Model file for the job. Use its own axes, mm. Face numbers are marked on the shaded views. A direction names the side the tool comes from. Coordinates: 2 decimals unless noted, no trailing zeros. Order: outer loops, then holes, each group sorted by start corner. A loop starts at its lowest first (then second) coordinate and runs counter-clockwise, first axis right, second up. Notation, with made-up numbers: (81, -27) -> (87, -27) arc R7 cw to (87, -17) -> close; hole circle Ø2 at (73.5, -14). An arc over 180 degrees is marked (long way). Return JSON: item names as keys, results as strings. Group by question number.
1) Which spindle directions (+Z, -Z, +X, -X, +Y, -Y) get a long thin tool onto all of the face, cutting with end or side? Do the marked faces 4 and 5. Say none if no direction does.
2) Cut at D-D (y = 73). Write the cut outline in (x, z), and give its area (3 significant figures).
3) Cut at B-B (x = 12). Write the cut outline in (y, z).
4) Pull direction Y, two halves, no side cores. Call the marked faces 1, 2 and 3: +Y half, -Y half, draft (parallel to the pull), parting line (faces both ways), or undercut.
5) Flat gauge pins, fed straight in: pin 1 (10 mm diameter, centred on y = 12, z = 16, fed in from -X); pin 2 (1 mm diameter, centred on x = 37.5, y = 57, fed in from -Z); pin 3 (5.5 mm diameter, centred on x = 11, y = 41.5, fed in from +Z). Where does each tip first touch, or does it go through?
6) Cut at A-A (z = 17.5). State how many separate pieces and enclosed holes the cut face has, and give its area (3 significant figures).
7) Probe line 1 (X direction, y = 26, z = 20.5); line 2 (Y direction, x = 53, z = 32.5); line 3 (X direction, y = 51.5, z = 6). List the from-to ranges inside material, lowest first.
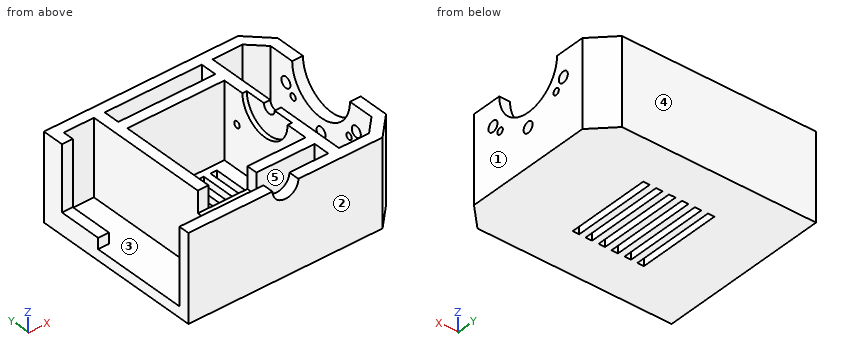
Autodesk Inventor part; units mm, degrees
ref_plane "YZ Plane" through (0, 0, 0) normal (1, 0, 0) x (0, 1, 0)
ref_plane "XZ Plane" through (0, 0, 0) normal (0, 1, 0) x (-1, 0, 0)
ref_plane "XY Plane" through (0, 0, 0) normal (0, 0, 1) x (1, 0, 0)
sketch "Sketch1" plane through (0, 0, 0) normal (0, 0, 1) x (1, 0, 0)
  line L0 (0, 0) -> (100, 0)
  line L1 (100, 0) -> (100, 80) construction
  line L2 (100, 80) -> (0, 80)
  line L3 (0, 80) -> (0, 0)
  line L4 (100, 70) -> (90, 80)
  line L5 (100, 10) -> (90, 0)
  line L6 (100, 70) -> (100, 10)
  line L7 (90, 0) -> (0, 0)
  line L8 (90, 80) -> (0, 80)
  dimension "d0" = 100
  dimension "d1" = 80
  dimension "d15" = 10
  dimension "d16" = 10
  dimension "d17" = 10
  dimension "d18" = 10
extrude "Extrusion1" add sketch "Sketch1" along normal blind 40
sketch "Sketch2" plane through (0, 0, 40) normal (0, 0, 1) x (1, 0, 0)
  line L0 (90, 80) -> (0, 80)
  line L1 (100, 70) -> (90, 80)
  line L2 (100, 10) -> (100, 70)
  line L3 (90, 0) -> (100, 10)
  line L4 (0, 0) -> (90, 0)
  line L5 (0, 75) -> (87.9289, 75)
  line L6 (87.9289, 75) -> (95, 67.9289)
  line L7 (95, 67.9289) -> (95, 12.0711)
  line L8 (95, 12.0711) -> (87.9289, 5)
  line L9 (87.9289, 5) -> (0, 5)
  line L10 (0, 80) -> (0, 0)
  line L11 (0, 75) -> (0, 5)
  dimension "d19" = 5
extrude "Extrusion2" cut sketch "Sketch2" against normal blind 35 contours L5 L6 L7 L8 L9 L10
sketch "Sketch3" plane through (0, 0, 0) normal (-1, 0, 0) x (0, 0, 1)
  line L0 (0, 80) -> (40, 80)
  line L1 (0, 0) -> (40, 0)
  line L2 (0, 80) -> (10, 80)
  line L3 (10, 80) -> (10, 50)
  line L4 (10, 50) -> (0, 50)
  line L5 (0, 50) -> (0, 80)
  line L6 (40, 80) -> (40, 0)
  line L7 (0, 80) -> (40, 80)
  line L8 (40, 80) -> (40, 70)
  line L9 (40, 70) -> (0, 70)
  line L10 (0, 70) -> (0, 80)
  line L11 (0, 0) -> (40, 0)
  line L12 (0, 80) -> (40, 80)
  point P0 (20, 0)
  point P1 (20, 80)
  dimension "d7" = 10
  dimension "d8" = 10
  dimension "d11" = 50
extrude "Extrusion3" add sketch "Sketch3" against normal blind 5
sketch "Sketch4" plane through (100, 10, 0) normal (1, 0, 0) x (0, 0, -1)
  circle A0 centre (-40, 30) radius 16
  line L0 (-40, 0) -> (-40, 60)
  point P0 (66.6667, -50)
  dimension "d12" = 32
extrude "Extrusion4" cut sketch "Sketch4" against normal through all
sketch "Sketch5" plane through (0, 0, 5) normal (0, 0, 1) x (1, 0, 0)
  line L0 (74, 75) -> (69, 75)
  line L1 (69, 75) -> (69, 5)
  line L2 (69, 5) -> (74, 5)
  line L3 (74, 5) -> (74, 75)
  line L4 (87.9289, 5) -> (0, 5)
  line L5 (5, 75) -> (87.9289, 75)
  line L6 (95, 67.9289) -> (95, 56)
  point P0 (0, 0)
  dimension "d20" = 5
  dimension "d21" = 21
extrude "Extrusion5" add sketch "Sketch5" along normal blind 35
sketch "Sketch6" plane through (69, 5, 5) normal (-1, 0, 0) x (0, 0, 1)
  line L0 (35, 70) -> (35, 0)
  circle A0 centre (35, 35) radius 3
  line L1 (19.5, 19.5) -> (50.5, 19.5) construction
  line L2 (50.5, 19.5) -> (50.5, 50.5) construction
  line L3 (50.5, 50.5) -> (19.5, 50.5) construction
  line L4 (19.5, 50.5) -> (19.5, 19.5) construction
  line L5 (19.5, 19.5) -> (50.5, 50.5) construction
  line L6 (50.5, 19.5) -> (19.5, 50.5) construction
  circle A1 centre (19.5, 50.5) radius 1.5
  circle A2 centre (19.5, 19.5) radius 1.5
  point P0 (-5, -5)
  dimension "d24" = 6
  dimension "d25" = 31
  dimension "d26" = 31
  dimension "d27" = 3
  dimension "d28" = 3
extrude "Extrusion6" cut sketch "Sketch6" against normal through all
sketch "Sketch7" plane through (69, 5, 5) normal (-1, 0, 0) x (0, 0, 1)
  arc A0 (35, 38) -> (35, 32) centre (35, 35) ccw
  circle A1 centre (35, 35) radius 12.5
  point P0 (-5, -5)
  dimension "d31" = 25
extrude "Extrusion7" cut sketch "Sketch7" against normal blind 2
sketch "Sketch8" plane through (0, 0, 5) normal (0, 0, 1) x (1, 0, 0)
  line L0 (69, 17.5) -> (19, 17.5)
  line L1 (19, 17.5) -> (19, 12.5)
  line L2 (19, 12.5) -> (69, 12.5)
  line L3 (69, 12.5) -> (69, 17.5)
  line L4 (69, 27.5) -> (69, 5)
  line L5 (69, 67.5) -> (19, 67.5)
  line L6 (19, 67.5) -> (19, 62.5)
  line L7 (19, 62.5) -> (69, 62.5)
  line L8 (69, 62.5) -> (69, 67.5)
  line L9 (19, 62.5) -> (19, 17.5) construction
  line L10 (69, 27.5) -> (69, 52.5) construction
  point P0 (0, 0)
  point P1 (69, 15)
  point P2 (19, 40)
  point P3 (69, 40)
  dimension "d34" = 50
  dimension "d35" = 5
  dimension "d36" = 50
  dimension "d37" = 5
  dimension "d38" = 45
extrude "Extrusion8" add sketch "Sketch8" along normal blind 35
sketch "Sketch9" plane through (0, 0, 5) normal (0, 0, 1) x (1, 0, 0)
  line L0 (19, 75) -> (24, 75)
  line L1 (24, 75) -> (24, 5)
  line L2 (24, 5) -> (19, 5)
  line L3 (19, 5) -> (19, 75)
  line L4 (5, 75) -> (69, 75)
  line L5 (69, 5) -> (0, 5)
  point P0 (0, 0)
  point P1 (19, 12.5)
  dimension "d41" = 5
extrude "Extrusion9" add sketch "Sketch9" along normal blind 35
sketch "Sketch10" plane through (0, 0, 40) normal (0, 0, 1) x (1, 0, 0)
  line L0 (24, 17.5) -> (69, 17.5)
  line L1 (19, 5) -> (19, 75)
  line L2 (42, 17.5) -> (19, 17.5)
  line L3 (19, 17.5) -> (19, 5)
  line L4 (19, 5) -> (42, 5)
  line L5 (42, 5) -> (42, 17.5)
  point P0 (0, 0)
  dimension "d44" = 23
extrude "Extrusion10" cut sketch "Sketch10" against normal blind 10
sketch "Sketch11" plane through (0, 0, 5) normal (0, 0, 1) x (1, 0, 0)
  line L0 (30, 59.5) -> (33, 59.5)
  line L1 (33, 59.5) -> (33, 20.5)
  line L2 (33, 20.5) -> (30, 20.5)
  line L3 (30, 20.5) -> (30, 59.5)
  line L4 (24, 62.5) -> (69, 62.5)
  line L5 (24, 17.5) -> (42, 17.5)
  line L6 (24, 17.5) -> (24, 62.5)
  line L7 (36, 59.5) -> (39, 59.5)
  line L8 (39, 59.5) -> (39, 20.5)
  line L9 (39, 20.5) -> (36, 20.5)
  line L10 (36, 20.5) -> (36, 59.5)
  line L11 (42, 59.5) -> (45, 59.5)
  line L12 (45, 59.5) -> (45, 20.5)
  line L13 (45, 20.5) -> (42, 20.5)
  line L14 (42, 20.5) -> (42, 59.5)
  line L15 (48, 59.5) -> (51, 59.5)
  line L16 (51, 59.5) -> (51, 20.5)
  line L17 (51, 20.5) -> (48, 20.5)
  line L18 (48, 20.5) -> (48, 59.5)
  line L19 (54, 59.5) -> (57, 59.5)
  line L20 (57, 59.5) -> (57, 20.5)
  line L21 (57, 20.5) -> (54, 20.5)
  line L22 (54, 20.5) -> (54, 59.5)
  line L23 (60, 59.5) -> (63, 59.5)
  line L24 (63, 59.5) -> (63, 20.5)
  line L25 (63, 20.5) -> (60, 20.5)
  line L26 (60, 20.5) -> (60, 59.5)
  point P0 (0, 0)
  dimension "d47" = 3
  dimension "d48" = 3
  dimension "d49" = 3
  dimension "d50" = 6
  dimension "d53" = 6
extrude "Extrusion11" cut sketch "Sketch11" against normal through all
sketch "Sketch12" plane through (0, 0, 0) normal (0, -1, 0) x (1, 0, 0)
  circle A0 centre (45, 40) radius 6
  line L0 (0, 40) -> (90, 40)
  point P0 (0, 0)
  dimension "d60" = 12
extrude "Extrusion12" cut sketch "Sketch12" against normal blind 5
sketch "Sketch13" plane through (100, 10, 0) normal (1, 0, 0) x (0, 0, -1)
  circle A0 centre (-17.5, 30) radius 2.5
  arc A1 (-40, 14) -> (-40, 46) centre (-40, 30) ccw
  circle A2 centre (-28.75, 49.4856) radius 2.5
  circle A3 centre (-51.25, 49.4856) radius 2.5
  circle A4 centre (-62.5, 30) radius 2.5
  circle A5 centre (-51.25, 10.5144) radius 2.5
  circle A6 centre (-28.75, 10.5144) radius 2.5
  point P0 (0, -10)
  dimension "d63" = 5
  dimension "d64" = 22.5
  dimension "d67" = 360
extrude "Extrusion13" cut sketch "Sketch13" against normal blind 10 contours A0 | A2 | A6
properties part number "FA001" material "ABS Plastic"
Answers below:
{
 "1": {"face 4": "+Z, -Z, +X, -X, +Y", "face 5": "+Z"},
 "2": {"outline": "(0, 0) -> (97, 0) -> (97, 40) -> (89.93, 40) -> (89.93, 5) -> (74, 5) -> (74, 40) -> (69, 40) -> (69, 5) -> (24, 5) -> (24, 40) -> (19, 40) -> (19, 5) -> (5, 5) -> (5, 40) -> (0, 40) -> close", "area": "1,260 mm^2"},
 "3": {"outline": "(0, 0) -> (80, 0) -> (80, 40) -> (75, 40) -> (75, 5) -> (5, 5) -> (5, 40) -> (0, 40) -> close"},
 "4": {"face 1": "draft", "face 2": "-Y half", "face 3": "undercut"},
 "5": {"pin 1": "stops at x = 19", "pin 2": "passes through", "pin 3": "stops at z = 5"},
 "6": {"separate pieces": "1", "enclosed holes": "3", "area": "2,450 mm^2"},
 "7": {"line 1": "x = 19 to 24, 69 to 74, 95 to 100", "line 2": "y = 0 to 5, 12.5 to 17.5, 62.5 to 67.5, 75 to 80", "line 3": "x = 0 to 5, 19 to 24, 69 to 74, 95 to 100"}
}
